from build123d import *

# Parameters (mm, degrees)
F0_W           = 65
F0_H           = 36
F0_R           = 11.5
F1_DEPTH       = 8
F3_D           = 3.3
F3_CBORE_D     = 6.5
F3_CBORE_DEPTH = 3
F4_SIZE        = 0.5
F6_D           = 2.5
F6_DEPTH       = 13.5
F6_TIP         = 0.7510757738
F7_W           = 36
F7_H           = 36
F7_R           = 1.65
F7_R_2         = 11.5
F8_DEPTH       = 2


with BuildPart() as f1:
    # F0 (on Front) → F1 (new body)
    with BuildSketch(Plane.XZ):
        Rectangle(F0_W, F0_H)
        Circle(F0_R, mode=Mode.SUBTRACT)
    extrude(amount=F1_DEPTH)

    # F3 (through all)
    with Locations(Plane.XZ.offset(8)):
        with Locations((13, 13), (13, -13), (-13, -13), (-13, 13)):
            CounterBoreHole(F3_D / 2, F3_CBORE_D / 2, F3_CBORE_DEPTH)

    # F4
    f4_edges = [f1.edges().sort_by_distance(p)[0] for p in [
        (-32.5, -4, 18),
        (32.5, -4, 18),
        (32.5, -4, -18),
        (-32.5, -4, -18),
    ]]
    chamfer(f4_edges, length=F4_SIZE)

    # F6
    with Locations(Plane(origin=(0, 0, -18), x_dir=(1, 0, 0), z_dir=(0, 0, -1))):
        with Locations((27, 4), (-27, 4)):
            Hole(F6_D / 2, depth=F6_DEPTH)
            with Locations((0, 0, -(F6_DEPTH + F6_TIP / 2))):  # 118° drill point
                Cone(0, F6_D / 2, F6_TIP, mode=Mode.SUBTRACT)

    # F7 (on face) → F8 (cut)
    with BuildSketch(Plane(origin=(0, 0, 0), x_dir=(-1, 0, 0), z_dir=(0, 1, 0))):
        Rectangle(F7_W, F7_H)
        with Locations((-13, -13)):
            Circle(F7_R, mode=Mode.SUBTRACT)
        with Locations((13, -13)):
            Circle(F7_R, mode=Mode.SUBTRACT)
        with Locations((-13, 13)):
            Circle(F7_R, mode=Mode.SUBTRACT)
        Circle(F7_R_2, mode=Mode.SUBTRACT)
        with Locations((13, 13)):
            Circle(F7_R, mode=Mode.SUBTRACT)
    extrude(amount=-F8_DEPTH, mode=Mode.SUBTRACT)


solid = f1.part
The model under review builds one solid part; all positions refer to its coordinate system, in mm. A direction names the side the tool comes from. Coordinates: 2 decimals unless noted, no trailing zeros. Loops run counter-clockwise (first coordinate to the right, second up) from the corner with the lowest first, then second, coordinate; pieces in that order, holes last. Notation, with made-up numbers: (55.5, -0.75) -> (79.5, -0.75) arc R34 cw to (79.5, 31.25) -> close; hole circle Ø9 at (59, 32). An arc over 180 degrees is marked (long way). Use a Markdown table: item, result. Add a question column.
1. Add section C-C on x = 13. Write out the cut boundary in (y, z), plus the area to 3 significant figures.
2. Add section D-D on x = 0. Write out the cut boundary in (y, z), plus the area to 3 significant figures.
3. Add section A-A on z = -13. Write out the cut boundary in (x, y), plus the area to 3 significant figures.
4. Draft analysis for pull direction Z (two halves, no side actions). For faces 5 (the face through (32.5, -4, 0)), 6 (the face through (0, -4, 18)), 7 (the face through (11.476, -3.479, 12.368)), 8 (the face through (27.2, -3.92, -3.88)), state which applies: pulls with the +Z half, pulls with the -Z half, needs draft (parallel to the pull), parting line crosses it, or undercut.
5. To check wall thickness, follow line 1 (Z direction, x = -13, y = -6.1); line 2 (X direction, y = -1.25, z = -8.5); line 3 (Y direction, x = -27, z = -14.75). State the ranges of each line that lie inside material, in increasing order.
6. Add section B-B on z = 0. Write out the cut boundary in (x, y).
7. Clearance check with flat-ended pins moving along their axes: pin 1 Ø2 at (x, z) = (12, 13) entering from -Y; pin 2 Ø11 at (x, z) = (-4, -8) entering from +Y; pin 3 Ø2.5 at (x, z) = (13, -13) entering from -Y. State where each tip first meets the part, or that it passes through.
8. Machinability: for faces 1 (the face through (25, 0, 0)), 2 (the face through (18, -1, 0)), 3 (the face through (25.845, -3.521, -11.156)), 4 (the face through (-11.6, -5, -14.4)), which of the approach directions +Z, -Z, +X, -X, +Y, -Y give a long, thin tool a straight path to every point of the face, cutting with its end or side? Answer none if there is none.
Returned:
| question | item | result |
|---|---|---|
| 1 | outline | (-8, -18) -> (-2, -18) -> (-2, -14.65) -> (-5, -14.65) -> (-5, -16.25) -> (-8, -16.25) -> close; (-8, -9.75) -> (-5, -9.75) -> (-5, -11.35) -> (-2, -11.35) -> (-2, 11.35) -> (-5, 11.35) -> (-5, 9.75) -> (-8, 9.75) -> close; (-8, 16.25) -> (-5, 16.25) -> (-5, 14.65) -> (-2, 14.65) -> (-2, 18) -> (-8, 18) -> close |
| 1 | area | 157 mm² |
| 2 | outline | (-8, -18) -> (-2, -18) -> (-2, -11.5) -> (-8, -11.5) -> close; (-8, 11.5) -> (-2, 11.5) -> (-2, 18) -> (-8, 18) -> close |
| 2 | area | 78.0 mm² |
| 3 | outline | (-32.5, -8) -> (-16.25, -8) -> (-16.25, -5) -> (-14.65, -5) -> (-14.65, -2) -> (-18, -2) -> (-18, 0) -> (-32.5, 0) -> close; (-11.35, -5) -> (-9.75, -5) -> (-9.75, -8) -> (9.75, -8) -> (9.75, -5) -> (11.35, -5) -> (11.35, -2) -> (-11.35, -2) -> close; (14.65, -5) -> (16.25, -5) -> (16.25, -8) -> (32.5, -8) -> (32.5, 0) -> (18, 0) -> (18, -2) -> (14.65, -2) -> close; hole circle Ø2.5 at (-27, -4); hole circle Ø2.5 at (27, -4) |
| 3 | area | 379 mm² |
| 4 | face 5 | needs draft |
| 4 | face 6 | pulls with the +Z half |
| 4 | face 7 | undercut |
| 4 | face 8 | pulls with the -Z half |
| 5 | line 1 | z = -18 to -16.25, -9.75 to 9.75, 16.25 to 18 |
| 5 | line 2 | x = -32.5 to -18, 18 to 32.5 |
| 5 | line 3 | y = -8 to -5.25, -2.75 to 0 |
| 6 | outline | (-32.5, -8) -> (-11.5, -8) -> (-11.5, -2) -> (-18, -2) -> (-18, 0) -> (-32.5, 0) -> close; (11.5, -8) -> (32.5, -8) -> (32.5, 0) -> (18, 0) -> (18, -2) -> (11.5, -2) -> close |
| 7 | pin 1 | stops at y = -5 |
| 7 | pin 2 | stops at y = -2 |
| 7 | pin 3 | passes through |
| 8 | face 1 | +Z, -Z, +X, -X, +Y |
| 8 | face 2 | +Z, -Z, +Y |
| 8 | face 3 | -Z |
| 8 | face 4 | -Y |
